Can you work these out from the drawing? Everything is in mm from the part's minimum corner. Coordinates: 2 decimals unless noted, no trailing zeros. Write each loop counter-clockwise with the first axis right and the second up, starting at its lowest first coordinate (ties: lowest second). Pieces come first, ordered by that corner, then holes. Notation, with made-up numbers: (5.25, 3.25) -> (48.25, 3.25) arc R9 ccw to (48.25, 9.25) -> close; hole circle Ø7 at (76, 13). An arc over 180 degrees is marked (long way). Answer as CSV lines item,"result". Start each with the question number.
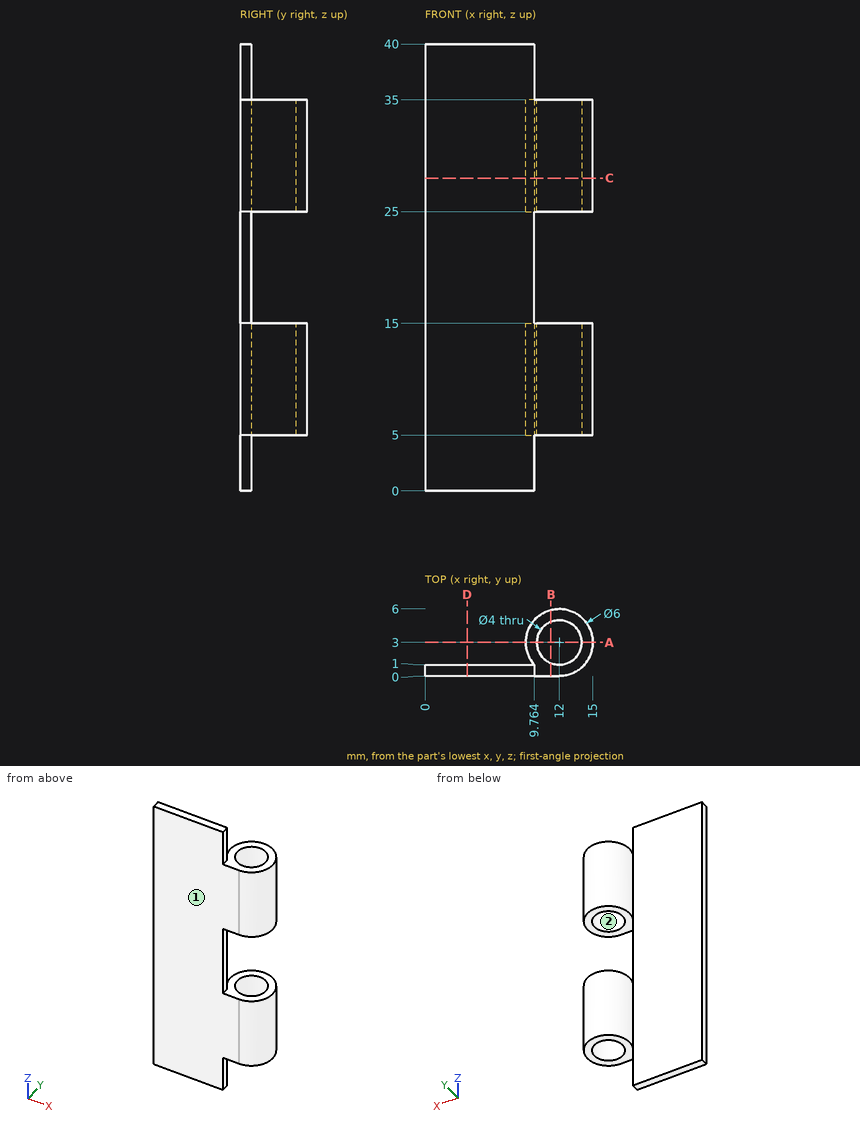
Q1. For pin 1 (2 mm diameter, centred on y = 5, z = 11, fed in from -X); pin 2 (5 mm diameter, centred on x = 7, z = 15, fed in from +Y); pin 3 (1.8 mm diameter, centred on x = 10.5, y = 3, fed in from +Z), each with a flat end and sliding along its axis, tell me the tip position at first contact or that it passes through.
Q2. If we mould it in two halves opening along Y, with no side actions, what happens to the marked faces 1 and 2? For each: released by +Y, released by -Y, zero draft, split by the parting line, or undercut.
Q3. I need wall thicknesses on L1, parallel to Z at x = 13, y = 5; L2, parallel to Y at x = 12, z = 28.5; L3, parallel to Y at x = 1.5, z = 29.5. Which ranges of each line are inside material? Lowest first, please.
Q4. Imagine slicing it at A-A (y = 3). Write out the boundary of the cut face in (x, z).
Q5. Imagine slicing it at B-B (x = 11.25). Write out the boundary of the cut face in (y, z).
Q6. Imagine slicing it at D-D (x = 3.75). Write out the boundary of the cut face in (y, z).
Q7. Imagine slicing it at C-C (z = 28). Write out the boundary of the cut face in (x, y).
Entries:
1,pin 1,"x = 9.17"
1,pin 2,"y = 4.66"
1,pin 3,"z = 35"
2,face 1,"released by -Y"
2,face 2,"undercut"
3,L1,"5 to 15, 25 to 35"
3,L2,"0 to 1, 5 to 6"
3,L3,"0 to 1"
4,outline,"(9, 5) -> (10, 5) -> (10, 15) -> (9, 15) -> close; (9, 25) -> (10, 25) -> (10, 35) -> (9, 35) -> close; (14, 5) -> (15, 5) -> (15, 15) -> (14, 15) -> close; (14, 25) -> (15, 25) -> (15, 35) -> (14, 35) -> close"
5,outline,"(0, 5) -> (1.15, 5) -> (1.15, 15) -> (0, 15) -> close; (0, 25) -> (1.15, 25) -> (1.15, 35) -> (0, 35) -> close; (4.85, 5) -> (5.9, 5) -> (5.9, 15) -> (4.85, 15) -> close; (4.85, 25) -> (5.9, 25) -> (5.9, 35) -> (4.85, 35) -> close"
6,outline,"(0, 0) -> (1, 0) -> (1, 40) -> (0, 40) -> close"
7,outline,"(0, 0) -> (12, 0) arc R3 ccw (long way) to (9.76, 1) -> (0, 1) -> close; hole circle Ø4 at (12, 3)"
